```python
from build123d import *

# Parameters (mm, degrees)
F0_W     = 40
F0_H     = 40
F1_DEPTH = 40
F2_DEPTH = 25


with BuildPart() as f1:
    # F0 (on Top) → F1 (new body)
    with BuildSketch(Plane.XY):
        Polygon((20, 20), (0, 0), (40, 0), align=None)
        with Locations((20, -20)):
            Rectangle(F0_W, F0_H)
    extrude(amount=F1_DEPTH)

    # F0 (on Top) → F2 (cut)
    with BuildSketch(Plane.XY):
        with Locations((20, -20)):
            Rectangle(F0_W, F0_H)
    extrude(amount=F2_DEPTH, mode=Mode.SUBTRACT)


solid = f1.part
```
Source: CAD feature listing. Evaluate the final solid. Frame: model axes, mm. A direction names the side the tool comes from. Give positions to 0.01 mm unless a question says otherwise; leave off trailing zeros. Loops run counter-clockwise (first coordinate to the right, second up) from the corner with the lowest first, then second, coordinate; pieces in that order, holes last. Notation, with made-up numbers: (78, 23.5) -> (136, 23.5) arc R9 ccw to (136, 27.5) -> close; hole circle Ø5 at (21.5, -9). An arc over 180 degrees is marked (long way). Put each result on its own line as item: value. Start each with the question number.
1) Cut plane B-B (z = 32.5). Return loops of the section in (x, y).
2) Reachability of faces 1 (the face through (40, -20, 32)), 2 (the face through (20, 0, 12)) from +Z, -Z, +X, -X, +Y, -Y: full face, straight path, thin tool, end or side. Return the list, or none.
3) Contact query for flat-ended pins moving along their axis: P1, Ø12, axis at y = -12.5, z = 15, coming from the -X side; P2, Ø12, axis at x = 29.5, y = -20, coming from the -Z side; P3, Ø12.5, axis at x = 28, z = 15, coming from the -Y side; P4, Ø8, axis at y = 13.5, z = 5, coming from the +X side. Output: stop coordinate, or through.
4) Cut plane A-A (x = 24.5). Return loops of the section in (y, z), then the cut area to 3 significant figures.
5) Material intervals for probe 1 along Z at (x, y) = (28, -8.5); probe 2 along Y at (x, z) = (23, 21); probe 3 along X at (y, z) = (10, 37.5), sorted ascending.
6) Cut plane C-C (y = -29.5). Return loops of the section in (x, z), then the cut area to 3 significant figures.
7) Cut plane D-D (x = 34.5). Return loops of the section in (y, z).
Results are:
1. outline: (0, -40) -> (40, -40) -> (40, 0) -> (20, 20) -> (0, 0) -> close
2. face 1: +Z, -Z, +X, +Y, -Y
2. face 2: -Z, +X, -X, -Y
3. P1: passes through
3. P2: stops at z = 25
3. P3: stops at y = 0
3. P4: stops at x = 30.5
4. outline: (-40, 25) -> (0, 25) -> (0, 0) -> (15.5, 0) -> (15.5, 40) -> (-40, 40) -> close
4. area: 1,220 mm2
5. probe 1: z = 25 to 40
5. probe 2: y = 0 to 17
5. probe 3: x = 10 to 30
6. outline: (0, 25) -> (40, 25) -> (40, 40) -> (0, 40) -> close
6. area: 600 mm2
7. outline: (-40, 25) -> (0, 25) -> (0, 0) -> (5.5, 0) -> (5.5, 40) -> (-40, 40) -> close
